Source: CAD feature listing. Evaluate the final solid. Frame: model axes, mm. A direction names the side the tool comes from. Give positions to 0.01 mm unless a question says otherwise; leave off trailing zeros. Order: outer loops, then holes, each group sorted by start corner. A loop starts at its lowest first (then second) coordinate and runs counter-clockwise, first axis right, second up. Notation, with made-up numbers: (74.5, 63.25) -> (82.5, 63.25) arc R17 ccw to (82.5, 95.25) -> close; hole circle Ø5 at (48, 16.25). An arc over 180 degrees is marked (long way). Answer in a Markdown table with one row per item.
```python
from build123d import *

# Parameters (mm, degrees)
F0_W     = 65
F0_H     = 20
F1_DEPTH = 8
F2_T     = -6
F4_DEPTH = 5


with BuildPart() as f1:
    # F0 (on Top) → F1 (new body)
    with BuildSketch(Plane.XY):
        Rectangle(F0_W, F0_H)
    extrude(amount=F1_DEPTH)

    # F2
    f2_openings = [f1.faces().sort_by_distance(p)[0] for p in [
        (0, 0, 8),
    ]]
    offset(amount=F2_T, openings=f2_openings)

    # F3 (on face) → F4 (join)
    with BuildSketch(Plane(origin=(0, 10, 0), x_dir=(-1, 0, 0), z_dir=(0, 1, 0))):
        with BuildLine():
            ThreePointArc((1.740197, 4), (1.230505, 5.230505), (0, 5.740197))
            Line((0, 5.740197), (0, 4))
            Line((0, 4), (0, 2.259803))
            ThreePointArc((0, 2.259803), (1.230505, 2.769495), (1.740197, 4))
        make_face()
        with BuildLine():
            Line((0, 4), (0, 5.740197))
            ThreePointArc((0, 5.740197), (-1.740197, 4), (0, 2.259803))
            Line((0, 2.259803), (0, 4))
        make_face()
    extrude(amount=F4_DEPTH)


solid = f1.part
```
(1) Section query B-B (y = 2). Return the cut outline in (x, z).
A:
| item | result |
|---|---|
| outline | (-32.5, 0) -> (32.5, 0) -> (32.5, 8) -> (26.5, 8) -> (26.5, 6) -> (-26.5, 6) -> (-26.5, 8) -> (-32.5, 8) -> close |
(2) Pull-direction query (X, two-part tool) for faces 3 (the flat face through (0, 5, 8)), 4 (the flat face through (0, -4, 7)), 5 (the flat face through (-32.5, 0, 4)), 6 (the flat face through (0, 0, 6)); classes: +X half, -X half, draft (parallel to the pull), parting line (faces both ways), or undercut.
A:
| item | result |
|---|---|
| face 3 | draft |
| face 4 | undercut |
| face 5 | -X half |
| face 6 | undercut |
(3) Access query for faces 1 (the flat face through (-26.5, 0, 7)), 2 (the flat face through (0, -10, 4)). Directions: +Z, -Z, +X, -X, +Y, -Y. A direction counts if a zero-diameter tool reaches every point of the face in a straight line with its end or side. Return the directions, or none.
A:
| item | result |
|---|---|
| face 1 | +Z |
| face 2 | +Z, -Z, +X, -X, -Y |
(4) Section query A-A (x = -5.5). Return the cut outline in (y, z), plus the area to 3 significant figures.
A:
| item | result |
|---|---|
| outline | (-10, 0) -> (10, 0) -> (10, 8) -> (4, 8) -> (4, 6) -> (-4, 6) -> (-4, 8) -> (-10, 8) -> close |
| area | 144 mm^2 |
(5) First-contact query: pin 1 Ø2 at (x, z) = (11, 7) entering from +Y; pin 2 Ø4 at (x, y) = (-4.5, 0.5) entering from +Z. Flat tips, straight axial feed; report the tip coordinate or a pass-through.
A:
| item | result |
|---|---|
| pin 1 | stops at y = 10 |
| pin 2 | stops at z = 6 |
(6) Ray query, probe 1 along X at (y, z) = (0.5, 6.5); probe 2 along Y at (x, z) = (2, 7.25); probe 3 along Y at (x, z) = (25, 5.5). Return the intervals inside material, ascending.
A:
| item | result |
|---|---|
| probe 1 | x = -32.5 to -26.5, 26.5 to 32.5 |
| probe 2 | y = -10 to -4, 4 to 10 |
| probe 3 | y = -10 to 10 |
(7) Section query C-C (y = 13.75). Return the cut outline in (x, z).
A:
| item | result |
|---|---|
| outline | circle Ø3.48 at (0, 4) |
